```python
from build123d import *

# Parameters (mm, degrees)
F0_R     = 1.6
F1_DEPTH = 1.5


# Not quite as in the source:
# - ends of sketch curves that miss each other by under 0.0002 mm in the source are joined


with BuildPart() as f1:
    # F0 (on Top) → F1 (new body)
    with BuildSketch(Plane.XY):
        with BuildLine():
            Line((-9.1814305153, -17.5127292487), (-6.6814305153, -17.5127292487))
            Line((-6.6814305153, -17.5127292487), (-5.1814305153, -16.0127292487))
            Line((-5.1814305153, -16.0127292487), (1.3185694847, -16.0127292487))
            Line((1.3185694847, -16.0127292487), (21.2185694847, -23.0127292487))
            Line((21.2185694847, -23.0127292487), (42.2185694847, -23.0127292487))
            Line((42.2185694847, -23.0127292487), (56.4220884847, -20.5127292487))
            Line((56.4220884847, -20.5127292487), (66.4220884847, -20.5127292487))
            ThreePointArc((66.4220884847, -20.5127292487), (74.8259566177, -17.2661070322), (78.864355153, -9.2127293132))
            Line((78.864355153, -9.2127293132), (78.8643544847, 18.1872707513))
            ThreePointArc((78.8643544847, 18.1872707513), (74.8259566177, 26.2406485347), (66.4220884847, 29.4872707513))
            Line((66.4220884847, 29.4872707513), (56.4220884847, 29.4872707513))
            Line((56.4220884847, 29.4872707513), (42.2185694847, 31.9872707513))
            Line((42.2185694847, 31.9872707513), (21.2185694847, 31.9872707513))
            Line((21.2185694847, 31.9872707513), (1.3185694847, 24.9872707513))
            Line((1.3185694847, 24.9872707513), (-5.1814305153, 24.9872707513))
            Line((-5.1814305153, 24.9872707513), (-6.6814305153, 26.4872707513))
            Line((-6.6814305153, 26.4872707513), (-9.1814305153, 26.4872707513))
            Line((-9.1814305153, 26.4872707513), (-11.6814305153, 26.4872707513))
            Line((-11.6814305153, 26.4872707513), (-13.1814305153, 24.9872707513))
            Line((-13.1814305153, 24.9872707513), (-60.9814305153, 24.9872707513))
            Line((-60.9814305153, 24.9872707513), (-62.4814305153, 26.4872707513))
            Line((-62.4814305153, 26.4872707513), (-64.9814305153, 26.4872707513))
            Line((-64.9814305153, 26.4872707513), (-67.4814305153, 26.4872707513))
            Line((-67.4814305153, 26.4872707513), (-68.9814305153, 24.9872707513))
            Line((-68.9814305153, 24.9872707513), (-75.4814305153, 24.9872707513))
            Line((-75.4814305153, 24.9872707513), (-96.4814305153, 31.9872707513))
            Line((-96.4814305153, 31.9872707513), (-116.4814305153, 31.9872707513))
            Line((-116.4814305153, 31.9872707513), (-124.4814305153, 31.9872707513))
            Line((-124.4814305153, 31.9872707513), (-126.4814305153, 28.9872707513))
            Line((-126.4814305153, 28.9872707513), (-126.4814305153, -20.0127292487))
            Line((-126.4814305153, -20.0127292487), (-124.4814305153, -23.0127292487))
            Line((-124.4814305153, -23.0127292487), (-116.4814305153, -23.0127292487))
            Line((-116.4814305153, -23.0127292487), (-96.4814305153, -23.0127292487))
            Line((-96.4814305153, -23.0127292487), (-75.4814305153, -16.0127292487))
            Line((-75.4814305153, -16.0127292487), (-68.9814305153, -16.0127292487))
            Line((-68.9814305153, -16.0127292487), (-67.4814305153, -17.5127292487))
            Line((-67.4814305153, -17.5127292487), (-64.9814305153, -17.5127292487))
            Line((-64.9814305153, -17.5127292487), (-62.4814305153, -17.5127292487))
            Line((-62.4814305153, -17.5127292487), (-60.9814305153, -16.0127292487))
            Line((-60.9814305153, -16.0127292487), (-13.1814305153, -16.0127292487))
            Line((-13.1814305153, -16.0127292487), (-11.6814305153, -17.5127292487))
            Line((-11.6814305153, -17.5127292487), (-9.1814305153, -17.5127292487))
        make_face()
        with Locations((-110.3480007641, -16.0127292487)):
            Circle(F0_R, mode=Mode.SUBTRACT)
        with Locations((-101.1275529865, -13.0127292487)):
            Circle(F0_R, mode=Mode.SUBTRACT)
        with Locations((-52.3314305153, -10.7627292487)):
            Circle(F0_R, mode=Mode.SUBTRACT)
        with Locations((-21.8314305153, -10.7627292487)):
            Circle(F0_R, mode=Mode.SUBTRACT)
        with Locations((25.8646919559, -13.0127292487)):
            Circle(F0_R, mode=Mode.SUBTRACT)
        with Locations((35.0851397335, -16.0127292487)):
            Circle(F0_R, mode=Mode.SUBTRACT)
        with Locations((63.8643544847, -8.2627292487)):
            Circle(F0_R, mode=Mode.SUBTRACT)
        with Locations((-101.1275529865, 21.9872707513)):
            Circle(F0_R, mode=Mode.SUBTRACT)
        with Locations((-110.3480007641, 24.9872707513)):
            Circle(F0_R, mode=Mode.SUBTRACT)
        with Locations((-52.3314305153, 19.7372707513)):
            Circle(F0_R, mode=Mode.SUBTRACT)
        with Locations((63.8643544847, 17.2372707513)):
            Circle(F0_R, mode=Mode.SUBTRACT)
        with Locations((-21.8314305153, 19.7372707513)):
            Circle(F0_R, mode=Mode.SUBTRACT)
        with Locations((25.8646919559, 21.9872707513)):
            Circle(F0_R, mode=Mode.SUBTRACT)
        with Locations((35.0851397335, 24.9872707513)):
            Circle(F0_R, mode=Mode.SUBTRACT)
    extrude(amount=F1_DEPTH)


solid = f1.part
```
The listing builds one solid part. Answer for the finished solid, in the listing's coordinates (mm). A direction names the side the tool comes from. Give positions to 0.01 mm unless a question says otherwise; leave off trailing zeros. Loops run counter-clockwise (first coordinate to the right, second up) from the corner with the lowest first, then second, coordinate; pieces in that order, holes last. Notation, with made-up numbers: (59, -2) - (107, -2) arc R22 cw to (107, 4) - close; hole circle Ø8 at (47.5, -17). An arc over 180 degrees is marked (long way). Return JSON: item names as keys, results as strings. Group by question number.
1. Which of the six approach directions +Z, -Z, +X, -X, +Y, -Y give full straight-line access (tool end or side, diameter ignored) to faces 1 (the flat face through (-86.128, -19.562, 0.74)), 2 (the flat face through (-85.834, 28.438, 0.74)), 3 (the cylindrical face through (-99.601, 22.468, 0.74))?
2. Determine the mould class of faces 4 (the flat face through (-25, 5, 0)), 5 (the cylindrical face through (74.921, 26.153, 0.74)), 6 (the flat face through (11.129, -19.464, 0.74)) for opening direction X: pulls with the +X half, pulls with the -X half, needs draft (parallel to the pull), parting line crosses it, or undercut.
3. Given pin 1 Ø0.8 at (x, z) = (-66, 0.5) entering from -Y; pin 2 Ø3 at (x, y) = (-52.33, 19.74) entering from +Z, each flat-ended and moving along its own axis, determine where each tip first touches the part or whether it passes through.
4. Straight lines are drawn through the part: line 1 (Y direction, x = -23, z = 0.6); line 2 (Y direction, x = -51, z = 1.2); line 3 (X direction, y = 19.5, z = 0.7). For each, find the intervals that lie inside material, in ascending order. Write a range as [from, to].
5. Find section A-A (x = -65.5). Write down the section's boundary in (y, z), then the cut area to 3 significant figures.
6. Find section C-C (x = -30). Write down the section's boundary in (y, z).
7. Find section B-B (z = 0.75). State how many separate pieces and enclosed holes the cut face has, then the cut area to 3 significant figures.
Verdict:
{
 "1": {"face 1": "+Z, -Z, -Y", "face 2": "+Z, -Z, +Y", "face 3": "+Z, -Z"},
 "2": {"face 4": "needs draft", "face 5": "pulls with the +X half", "face 6": "undercut"},
 "3": {"pin 1": "stops at y = -17.51", "pin 2": "passes through"},
 "4": {"line 1": "y = [-16.01, -11.86], [-9.67, 18.64], [20.83, 24.99]", "line 2": "y = [-16.01, -11.65], [-9.88, 18.85], [20.62, 24.99]", "line 3": "x = [-126.48, -53.91], [-50.75, -23.41], [-20.25, 78.67]"},
 "5": {"outline": "(-17.51, 0) - (26.49, 0) - (26.49, 1.5) - (-17.51, 1.5) - close", "area": "66.0 mm^2"},
 "6": {"outline": "(-16.01, 0) - (24.99, 0) - (24.99, 1.5) - (-16.01, 1.5) - close"},
 "7": {"separate pieces": "1", "enclosed holes": "14", "area": "9,640 mm^2"}
}
